Could you check a few things on this model? Use its own coordinates, in mm. Coordinates: 2 decimals unless noted, no trailing zeros. Loops run counter-clockwise (first coordinate to the right, second up) from the corner with the lowest first, then second, coordinate; pieces in that order, holes last. Notation, with made-up numbers: M -10.5,19.5 L 19.5,19.5 A10 ccw 19.5,28.5 Z; hole C 53.5,56 d10. An arc over 180 degrees is marked long. Write each question's results on one line, items separated by ' | '.
```python
from build123d import *

# Parameters (mm, degrees)
SKETCH1_R               = 11
BOSS_EXTRUDE1_DEPTH     = 6.35
CUT_EXTRUDE1_DEPTH      = 383.821165724
CUT_EXTRUDE1_DEPTH_BACK = 383.821165724
SKETCH2_R               = 0.635


with BuildPart() as part:
    # Sketch1 → Boss-Extrude1 (new body)
    with BuildSketch(Plane.XY):
        with BuildLine():
            Line((54.2, -30.213113696), (80.87, -30.213113696))
            Line((80.87, -30.213113696), (290.352370469, -49.325))
            ThreePointArc((290.352370469, -49.325), (337.438235998, -41.792944501), (375.172105998, -12.638774172))
            ThreePointArc((375.172105998, -12.638774172), (377.448393763, 8.996243247), (359, 20.525))
            Line((359, 20.525), (54.2, 20.525))
            Line((54.2, 20.525), (54.2, -30.213113696))
        make_face()
        with Locations((359, 0)):
            Circle(SKETCH1_R, mode=Mode.SUBTRACT)
    extrude(amount=BOSS_EXTRUDE1_DEPTH)

    # Sketch2 → Cut-Extrude1 (cut, two sides: drawn at the far end of the back side and taken through both)
    with BuildSketch(Plane(origin=(0, 0, 0), x_dir=(-1, 0, 0), z_dir=(0, 0, -1)).offset(-CUT_EXTRUDE1_DEPTH_BACK)):
        with Locations((-70.71, -23.132056848)):
            Circle(SKETCH2_R)
        with Locations((-70.71, -4.844056848)):
            Circle(SKETCH2_R)
        with Locations((-70.71, 13.443943152)):
            Circle(SKETCH2_R)
    extrude(amount=CUT_EXTRUDE1_DEPTH + CUT_EXTRUDE1_DEPTH_BACK, mode=Mode.SUBTRACT)


solid = part.part
```
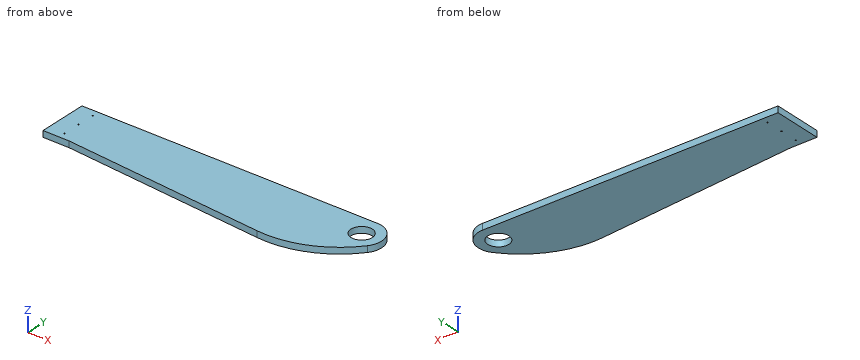
(1) Please list where these lines run through material, in increasing order: probe 1 along Y at (x, z) = (70.71, 2) (3 decimals); probe 2 along Y at (x, z) = (359, 4.25) (3 decimals); probe 3 along X at (y, z) = (13.5, 2.25). Write a range as from..to.
Reported:
probe 1: y = -30.213..-23.767, -22.497..-5.479, -4.209..12.809, 14.079..20.525 | probe 2: y = -28.906..-11, 11..20.525 | probe 3: x = 54.2..70.08, 71.34..374.46
(2) Imagine slicing it at A-A, the plane z = 4.5. List the corners of the cut face in (x, y) for me (3 decimals), and give its area (3 significant figures).
Reported:
outline: M 54.2,-30.213 L 80.87,-30.213 L 290.352,-49.325 A96.52 ccw 375.172,-12.639 A20.525 ccw 359,20.525 L 54.2,20.525 Z; hole C 70.71,-23.132 d1.27; hole C 70.71,-4.844 d1.27; hole C 70.71,13.444 d1.27; hole C 359,0 d22 | area: 18,700 mm2
(3) Imagine slicing it at B-B, the plane x = 239. List the corners of the cut face in (y, z) for me (3 decimals), and give its area (3 significant figures).
Reported:
outline: M -44.64,0 L 20.525,0 L 20.525,6.35 L -44.64,6.35 Z | area: 414 mm2
(4) Imagine slicing it at C-C, the plane y = -33.5. List the corners of the cut face in (x, z) for me, and give its area (3 significant figures).
Reported:
outline: M 116.9,0 L 352.68,0 L 352.68,6.35 L 116.9,6.35 Z | area: 1,500 mm2
(5) Will these pins go through, and if not, where does the flat tip stop? P1, Ø1, axis at x = 70.71, y = -4.84, coming from the +Z side; P2, Ø3, axis at y = -26.5, z = 5.5, coming from the +X side; P3, Ø1.9, axis at x = 69, z = 3, coming from the -Y side; P4, Ø1, axis at y = -33, z = 2, coming from the +X side.
Reported:
P1: passes through | P2: stops at x = 363.63 | P3: stops at y = -30.21 | P4: stops at x = 354.15
